```python
from build123d import *

# Parameters (mm, degrees)
F0_R      = 11.4211526137
F1_DEPTH  = 5.08
F3_R      = 19.685
F4_DEPTH  = 40.894
F6_DEPTH  = 5.08
F9_R      = 24.765
F10_DEPTH = 8.5
F11_R     = 13.97
F12_DEPTH = 12.7
F15_DEPTH = 31.75


with BuildPart() as f1:
    # F0 (on Front) → F1 (new body)
    with BuildSketch(Plane.XZ):
        Circle(F0_R)
    extrude(amount=F1_DEPTH)



with BuildPart() as f4:
    # F3 (on offset) → F4 (new body)
    with BuildSketch(Plane.YZ.offset(-15.5)):
        with Locations((-18, 0)):
            Circle(F3_R)
    extrude(amount=-F4_DEPTH)


with BuildPart() as f1_1:
    add(f1.part)

    add(f4.part)  # F6 merges F4
    # F5 (on face) → F6 (join, through all)
    with BuildSketch(Plane(origin=(0, 0, 0), x_dir=(-1, 0, 0), z_dir=(0, 1, 0))):
        with BuildLine():
            Line((19.05, 11.4211526137), (0, 11.4211526137))
            ThreePointArc((0, 11.4211526137), (8.0759744621, 8.0759744621), (11.4211526137, 0))
            ThreePointArc((11.4211526137, 0), (8.0759744621, -8.0759744621), (0, -11.4211526137))
            Line((0, -11.4211526137), (19.05, -11.4211526137))
            Line((19.05, -11.4211526137), (19.05, 11.4211526137))
        make_face()
    extrude(amount=-F6_DEPTH)

    # F9 (on face) → F10 (join)
    with BuildSketch(Plane(origin=(-56.394, 0, 0), x_dir=(0, -1, 0), z_dir=(-1, 0, 0))):
        with Locations((18, 0)):
            Circle(F9_R)
    extrude(amount=-F10_DEPTH)

    # F11 (on face) → F12 (join)
    with BuildSketch(Plane(origin=(-56.394, 0, 0), x_dir=(0, -1, 0), z_dir=(-1, 0, 0))):
        with Locations((18, 0)):
            Circle(F11_R)
    extrude(amount=F12_DEPTH)

    # F14 (on offset) → F15 (join)
    with BuildSketch(Plane.XZ.offset(22.5)):
        with BuildLine():
            ThreePointArc((-75.5499063227, 0), (-70.8743650094, 3.472069535), (-69.094, 9.017))
            ThreePointArc((-69.094, 9.017), (-69.2170356699, 10.5430051561), (-69.5829641441, 12.0295870961))
            Line((-69.5829641441, 12.0295870961), (-78.619, 12.0295870961))
            Line((-78.619, 12.0295870961), (-78.619, 0.508))
            ThreePointArc((-78.619, 0.508), (-77.0635740133, 0.3801418527), (-75.5499063227, 0))
        make_face()
        with BuildLine():
            Line((-69.094, -9.017), (-69.094, 9.017))
            ThreePointArc((-69.094, 9.017), (-70.8743650094, 3.472069535), (-75.5499063227, 0))
            ThreePointArc((-75.5499063227, 0), (-70.8743650094, -3.472069535), (-69.094, -9.017))
        make_face()
        with BuildLine():
            ThreePointArc((-69.5829641441, 12.0295870961), (-69.2170356699, 10.5430051561), (-69.094, 9.017))
            Line((-69.094, 9.017), (-69.094, 12.0295870961))
            Line((-69.094, 12.0295870961), (-69.5829641441, 12.0295870961))
        make_face()
        with BuildLine():
            Line((-78.619, 12.0295870961), (-69.5829641441, 12.0295870961))
            ThreePointArc((-69.5829641441, 12.0295870961), (-85.3330778344, 15.7732403624), (-81.6880936773, 0))
            ThreePointArc((-81.6880936773, 0), (-80.1744259867, 0.3801418527), (-78.619, 0.508))
            Line((-78.619, 0.508), (-78.619, 12.0295870961))
        make_face()
        with BuildLine():
            ThreePointArc((-69.094, -9.017), (-70.8743650094, -3.472069535), (-75.5499063227, 0))
            ThreePointArc((-75.5499063227, 0), (-77.0635740133, -0.3801418527), (-78.619, -0.508))
            Line((-78.619, -0.508), (-78.619, -12.0295870961))
            Line((-78.619, -12.0295870961), (-69.5829641441, -12.0295870961))
            ThreePointArc((-69.5829641441, -12.0295870961), (-69.2170356699, -10.5430051561), (-69.094, -9.017))
        make_face()
        with BuildLine():
            Line((-69.094, -12.0295870961), (-69.094, -9.017))
            ThreePointArc((-69.094, -9.017), (-69.2170356699, -10.5430051561), (-69.5829641441, -12.0295870961))
            Line((-69.5829641441, -12.0295870961), (-69.094, -12.0295870961))
        make_face()
        with BuildLine():
            ThreePointArc((-78.619, 0.508), (-80.1744259867, 0.3801418527), (-81.6880936773, 0))
            ThreePointArc((-81.6880936773, 0), (-80.1744259867, -0.3801418527), (-78.619, -0.508))
            Line((-78.619, -0.508), (-78.619, 0.508))
        make_face()
        with BuildLine():
            ThreePointArc((-78.619, -0.508), (-80.1744259867, -0.3801418527), (-81.6880936773, 0))
            ThreePointArc((-81.6880936773, 0), (-85.3330778344, -15.7732403624), (-69.5829641441, -12.0295870961))
            Line((-69.5829641441, -12.0295870961), (-78.619, -12.0295870961))
            Line((-78.619, -12.0295870961), (-78.619, -0.508))
        make_face()
    extrude(amount=-F15_DEPTH)


solid = f1_1.part
```
Input: part model. Units: mm. Frame: model coordinates. A direction names the side the tool comes from. Give positions to 0.01 mm unless a question says otherwise; leave off trailing zeros. Write each loop counter-clockwise with the first axis right and the second up, starting at its lowest first coordinate (ties: lowest second). Pieces come first, ordered by that corner, then holes. Notation, with made-up numbers: (41, 39.5) - (59, 39.5) arc R20 ccw to (59, 48.5) - close; hole circle Ø3 at (43.25, -10). An arc over 180 degrees is marked (long way). Write item = value, one per line. Start each with the question number.
1. Section query B-B, the plane y = -26. Output: boundary loops of the cut face in (x, z), then the cut area to 3 significant figures.
2. First-contact query: pin 1 Ø2.5 at (x, y) = (-8, -1.5) entering from -Z; pin 2 Ø7 at (x, z) = (-10.5, -3.5) entering from +Y; pin 3 Ø0.5 at (y, z) = (-10.5, 0) entering from +X. Flat tips, straight axial feed; report the tip coordinate or a pass-through.
3. Ray query, L1, parallel to X at y = -23.5, z = -1; L2, parallel to X at y = -27, z = 19.5; L3, parallel to X at y = -11, z = -12.5. Return the intervals inside material, ascending.
4. Section query D-D, the plane x = -32. Output: boundary loops of the cut face in (y, z) (3 decimals), then the cut area to 3 significant figures.
5. Access query for faces 4 (the flat face through (-2, -5.08, 0)), 5 (the flat face through (-56.394, -29, -11)), 6 (the flat face through (-19.05, -0.5, 10.4)). Directions: +Z, -Z, +X, -X, +Y, -Y. A direction counts if a zero-diameter tool reaches every point of the face in a straight line with its end or side. Return the directions, or none.
6. Section query A-A, the plane y = -18. Output: boundary loops of the cut face in (x, z) (3 decimals), then the cut area to 3 significant figures.
7. Section query C-C, the plane z = -10. Output: boundary loops of the cut face in (x, y).
8. Mould query, pull axis Z, two halves, no side actions, for faces 1 (the cylindrical face through (-77.042, -6.847, -0.377)), 2 (the flat face through (-9, -3, -11.421)), 3 (the flat face through (-79, 9.25, 0)). Classes: released by +Z, released by -Z, zero draft, split by the parting line, or undercut.
Check sheet entries:
q1.outline = (-69.09, -11.45) - (-56.39, -11.45) - (-56.39, -23.44) - (-47.89, -23.44) - (-47.89, -17.99) - (-15.5, -17.99) - (-15.5, 17.99) - (-47.89, 17.99) - (-47.89, 23.44) - (-56.39, 23.44) - (-56.39, 11.45) - (-69.09, 11.45) - close
q1.area = 1,850 mm2
q2.pin_1 = -11.42
q2.pin_2 = 0
q2.pin_3 = -15.5
q3.L1 = -69.09 to -15.5
q3.L2 = -56.39 to -47.89
q3.L3 = -87.48 to -69.75, -56.39 to -15.5
q4.outline = circle Ø39.37 at (-18, 0)
q4.area = 1,220 mm2
q5.face_4 = +Z, -Z, +X, -Y
q5.face_5 = none
q5.face_6 = +Z, +Y
q6.outline = (-81.688, 0) arc R9.525 ccw (long way) to (-69.583, -12.03) - (-69.094, -12.03) - (-69.094, -13.97) - (-56.394, -13.97) - (-56.394, -24.765) - (-47.894, -24.765) - (-47.894, -19.685) - (-15.5, -19.685) - (-15.5, 19.685) - (-47.894, 19.685) - (-47.894, 24.765) - (-56.394, 24.765) - (-56.394, 13.97) - (-69.094, 13.97) - (-69.094, 12.03) - (-69.583, 12.03) arc R9.525 ccw (long way) to start; hole (-78.619, -0.508) arc R9.525 ccw to (-75.55, 0) arc R9.525 ccw to (-78.619, 0.508) - close
q6.area = 2,650 mm2
q7.outline = (-88.09, -22.5) - (-69.09, -22.5) - (-69.09, -27.76) - (-56.39, -27.76) - (-56.39, -40.66) - (-47.89, -40.66) - (-47.89, -34.96) - (-15.5, -34.96) - (-15.5, -5.08) - (5.52, -5.08) - (5.52, 0) - (-19.05, 0) - (-19.05, -1.04) - (-47.89, -1.04) - (-47.89, 4.66) - (-56.39, 4.66) - (-56.39, -8.24) - (-69.09, -8.24) - (-69.09, 9.25) - (-88.09, 9.25) - close
q8.face_1 = undercut
q8.face_2 = released by -Z
q8.face_3 = zero draft
